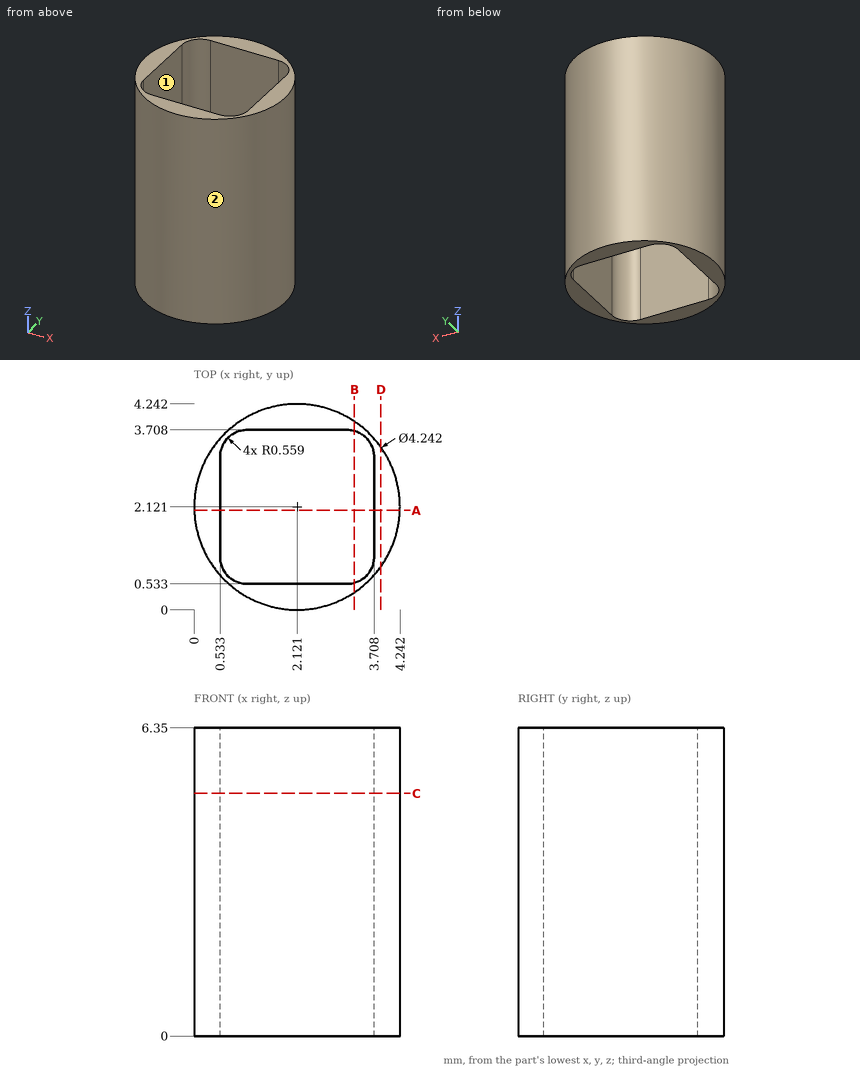
Here's the drawing with two shaded views (mm, measured from the low corner). I have some questions. Coordinates: 2 decimals unless noted, no trailing zeros. Loops run counter-clockwise (first coordinate to the right, second up) from the corner with the lowest first, then second, coordinate; pieces in that order, holes last. Notation, with made-up numbers: M 61.5,-35 L 85.5,-35 A28 ccw 85.5,-6 Z; hole C -19.5,-9.5 d8. An arc over 180 degrees is marked long. Answer as CSV lines item,"result". Start each with the question number.
1. For pin 1 Ø2 at (y, z) = (4, 4) entering from +X; pin 2 Ø2 at (x, z) = (0.5, 1.5) entering from -Y, each with a flat end and sliding along its axis, tell me the tip position at first contact or that it passes through.
2. Suppose I cut it at C-C, the plane z = 5. List the corners of the cut face in (x, y) for me.
3. Thinking about a two-plate mould opening in X: for the marked faces 1 and 2, which applies, +X half, -X half, draft (parallel to the pull), parting line (faces both ways), or undercut?
4. Suppose I cut it at A-A, the plane y = 2.05. List the corners of the cut face in (x, z) for me.
5. If I drill on probe 1 along X at (y, z) = (2.05, 4); probe 2 along Y at (x, z) = (2.95, 2.75), over which ranges is the centre line in solid material (lowest first)? Write a range as [from, to].
6. Suppose I cut it at D-D, the plane x = 3.85. List the corners of the cut face in (y, z) for me.
7. Suppose I cut it at B-B, the plane x = 3.3. List the corners of the cut face in (y, z) for me.
Output:
1,pin 1,"stops at x = 4.05"
1,pin 2,"stops at y = 0.09"
2,outline,"C 2.12,2.12 d4.24; hole M 0.53,1.09 A0.56 ccw 1.09,0.53 L 3.15,0.53 A0.56 ccw 3.71,1.09 L 3.71,3.15 A0.56 ccw 3.15,3.71 L 1.09,3.71 A0.56 ccw 0.53,3.15 Z"
3,face 1,"undercut"
3,face 2,"parting line"
4,outline,"M 0,0 L 0.53,0 L 0.53,6.35 L 0,6.35 Z; M 3.71,0 L 4.24,0 L 4.24,6.35 L 3.71,6.35 Z"
5,probe 1,"x = [0, 0.53], [3.71, 4.24]"
5,probe 2,"y = [0.17, 0.53], [3.71, 4.07]"
6,outline,"M 0.89,0 L 3.35,0 L 3.35,6.35 L 0.89,6.35 Z"
7,outline,"M 0.36,0 L 0.55,0 L 0.55,6.35 L 0.36,6.35 Z; M 3.69,0 L 3.88,0 L 3.88,6.35 L 3.69,6.35 Z"
